```python
from build123d import *

# Parameters (mm, degrees)
SKETCH2_W               = 84
SKETCH2_H               = 115
BOSS_EXTRUDE1_DEPTH     = 15
SKETCH3_W               = 15.5
SKETCH3_H               = 5
CUT_EXTRUDE1_DEPTH      = 144.199162009
MIRROR2_COPY_1_SKETCH_W = 15.5
MIRROR2_COPY_1_SKETCH_H = 5
MIRROR2_COPY_1_DEPTH    = 144.199162009
SKETCH4_W               = 53
SKETCH4_H               = 115
BOSS_EXTRUDE2_DEPTH     = 1


with BuildPart() as part:
    # Sketch2 → Boss-Extrude1 (new body)
    with BuildSketch(Plane.XY):
        with Locations((42, 57.5)):
            Rectangle(SKETCH2_W, SKETCH2_H)
    extrude(amount=BOSS_EXTRUDE1_DEPTH)

    # Sketch3 → Cut-Extrude1 (cut, through all)
    with BuildSketch(Plane(origin=(0, 115, 0), x_dir=(1, 0, 0), z_dir=(0, 1, 0))):
        with Locations((7.75, -12.5)):
            Rectangle(SKETCH3_W, SKETCH3_H)
    cut_extrude1 = extrude(amount=-CUT_EXTRUDE1_DEPTH, mode=Mode.SUBTRACT)

    # Mirror1: Cut-Extrude1 across plane
    add(cut_extrude1.mirror(Plane.XY.offset(7.5)), mode=Mode.SUBTRACT)

    # Mirror2: Cut-Extrude1 across plane
    add(cut_extrude1.mirror(Plane.ZY.offset(-42)), mode=Mode.SUBTRACT)

    # Mirror2 copy 1 sketch → Mirror2 copy 1 (cut, through all)
    with BuildSketch(Plane(origin=(84, 115, 15), x_dir=(-1, 0, 0), z_dir=(0, 1, 0))):
        with Locations((7.75, -12.5)):
            Rectangle(MIRROR2_COPY_1_SKETCH_W, MIRROR2_COPY_1_SKETCH_H)
    extrude(amount=-MIRROR2_COPY_1_DEPTH, mode=Mode.SUBTRACT)

    # Sketch4 → Boss-Extrude2 (add)
    with BuildSketch(Plane.XY.offset(15)):
        with Locations((42, 57.5)):
            Rectangle(SKETCH4_W, SKETCH4_H)
    extrude(amount=BOSS_EXTRUDE2_DEPTH)


solid = part.part
```
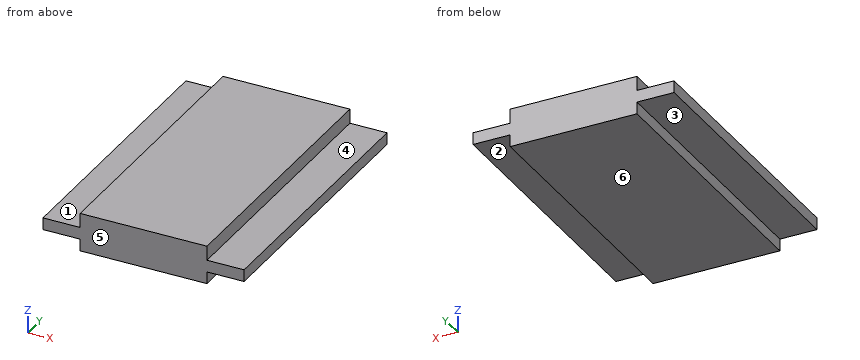
The listing builds one solid part. Answer for the finished solid, in the listing's coordinates (mm). Face numbers are marked on the shaded views. A direction names the side the tool comes from. Give positions to 0.01 mm unless a question says otherwise; leave off trailing zeros. Order: outer loops, then holes, each group sorted by start corner. A loop starts at its lowest first (then second) coordinate and runs counter-clockwise, first axis right, second up. Notation, with made-up numbers: (-7, -22.75) - (48, -22.75) arc R29 ccw to (48, -2.75) - close; hole circle Ø10 at (49.5, 33.25). An arc over 180 degrees is marked (long way). Answer in a Markdown table with one row per item. Add a question column.
Q1. Which of the six approach directions +Z, -Z, +X, -X, +Y, -Y give full straight-line access (tool end or side, diameter ignored) to the marked faces 1, 2 and 3?
Q2. Find the intervals of material crossed by line 1 along Z through (x, y) = (8, 28.5); line 2 along X through (y, z) = (50, 3.25), in increasing order. Write a range as [from, to].
Q3. Given P1, Ø4.5, axis at x = 78.5, y = 77.5, coming from the +Z side; P2, Ø1.5, axis at y = 32, z = 1.5, coming from the -X side; P3, Ø12.5, axis at x = 9, y = 56.5, coming from the -Z side, each flat-ended and moving along its own axis, determine where each tip first touches the part or whether it passes through.
Q4. The part is cut by section A-A (y = 17). Determine the outline of the cut face in (x, z), then the cut area to 3 significant figures.
Q5. The part is cut by section B-B (x = 75.5). Determine the outline of the cut face in (y, z).
Q6. The part is cut by section C-C (z = 1.5). Determine the outline of the cut face in (x, y), then the cut area to 4 significant figures.
Q7. For a pull along Z with two mould halves and no side action, classify the marked faces 4, 5 and 6 as released by +Z, released by -Z, zero draft, split by the parting line, or undercut.
Determined:
| question | item | result |
|---|---|---|
| 1 | face 1 | +Z, -X, +Y, -Y |
| 1 | face 2 | -Z, +X, +Y, -Y |
| 1 | face 3 | -Z, -X, +Y, -Y |
| 2 | line 1 | z = [5, 10] |
| 2 | line 2 | x = [15.5, 68.5] |
| 3 | P1 | stops at z = 10 |
| 3 | P2 | stops at x = 15.5 |
| 3 | P3 | stops at z = 5 |
| 4 | outline | (0, 5) - (15.5, 5) - (15.5, 0) - (68.5, 0) - (68.5, 5) - (84, 5) - (84, 10) - (68.5, 10) - (68.5, 16) - (15.5, 16) - (15.5, 10) - (0, 10) - close |
| 4 | area | 1,000 mm² |
| 5 | outline | (0, 5) - (115, 5) - (115, 10) - (0, 10) - close |
| 6 | outline | (15.5, 0) - (68.5, 0) - (68.5, 115) - (15.5, 115) - close |
| 6 | area | 6,095 mm² |
| 7 | face 4 | released by +Z |
| 7 | face 5 | zero draft |
| 7 | face 6 | released by -Z |
